Autodesk Inventor part; units mm, degrees
ref_plane "YZ Plane" through (0, 0, 0) normal (1, 0, 0) x (0, 1, 0)
ref_plane "XZ Plane" through (0, 0, 0) normal (0, 1, 0) x (-1, 0, 0)
ref_plane "XY Plane" through (0, 0, 0) normal (0, 0, 1) x (1, 0, 0)
sketch "Sketch1" plane through (0, 0, 0) normal (0, 0, 1) x (1, 0, 0)
  line L0 (-23.6137, 0) -> (-23.6137, 203.2)
  line L1 (-23.6137, 203.2) -> (484.3863, 203.2)
  line L2 (484.3863, 203.2) -> (484.3863, 279.4)
  line L3 (484.3863, 279.4) -> (1500.3863, 279.4)
  line L4 (1500.3863, 279.4) -> (1500.3863, 203.2)
  line L5 (1500.3863, 203.2) -> (2008.3863, 203.2)
  line L6 (2008.3863, 203.2) -> (2008.3863, 0)
  line L7 (2008.3863, 0) -> (-23.6137, 0)
  point P0 (0, 0)
  dimension "d0" = 203.2
  dimension "d1" = 508
  dimension "d2" = 76.2
  dimension "d3" = 1016
  dimension "d4" = 76.2
  dimension "d5" = 508
revolve "Revolution1" add sketch "Sketch1" angle 360 about axis through (2008.3863, 0, 0) along (-1, 0, 0)
chamfer "Chamfer1" distance 50.8 angle 45 2 edges at (-23.6137, -203.2, 0) (2008.3863, -203.2, 0)
properties part number "axle"
Work out the finished part from the listing and answer in its coordinate system (mm). A direction names the side the tool comes from. Coordinates: 2 decimals unless noted, no trailing zeros. Write each loop counter-clockwise with the first axis right and the second up, starting at its lowest first coordinate (ties: lowest second). Pieces come first, ordered by that corner, then holes. Notation, with made-up numbers: M 88,53 L 121,53 A16 cw 121,83 Z; hole C 44.25,80 d5. An arc over 180 degrees is marked long. Use one line per item in the form item = value. Start each with the question number.
1. The part is cut by section D-D (x = 897.5). Give the vertices of the cut face in (y, z).
2. Each of these flat-tipped pins is pushed along its axis until it touches: P1, Ø1.5, axis at x = 563, z = -153.5, coming from the +Y side; P2, Ø2, axis at y = -40, z = -207, coming from the -X side; P3, Ø8, axis at y = 64.5, z = -173.5, coming from the -X side. Where does it stop, or does it pass through?
3. Straight lines are drawn through the part: probe 1 along X at (y, z) = (-227.5, 116); probe 2 along X at (y, z) = (39, -170); probe 3 along Y at (x, z) = (1513.5, -188). For each, find the intervals that lie inside material, in ascending order. Write a range as from..to.
4. The part is cut by section C-C (x = 214). Give the vertices of the cut face in (y, z), plus the area to 3 significant figures.
5. The part is cut by section A-A (z = 0). Give the vertices of the cut face in (x, y), plus the area to 3 significant figures.
6. A tool of negligible diameter and unlimited length cuts with its end or side. For faces 1 (the face through (-23.614, -2, -2)), 2 (the face through (1732.187, -44.05, -198.368)), 3 (the face through (258.987, -44.05, -198.368)), from which of +Z, -Z, +X, -X, +Y, -Y can it reach the whole face along a straight path? Write none if from no direction.
Evaluation:
q1.outline = C 0,0 d558.8
q2.P1 = 233.95
q2.P2 = 484.39
q2.P3 = 5.09
q3.probe_1 = 484.39..1500.39
q3.probe_2 = -1.6..1986.37
q3.probe_3 = -77.11..77.11
q4.outline = C 0,0 d406.4
q4.area = 130,000 mm^2
q5.outline = M -23.61,-152.4 L 27.19,-203.2 L 484.39,-203.2 L 484.39,-279.4 L 1500.39,-279.4 L 1500.39,-203.2 L 1957.59,-203.2 L 2008.39,-152.4 L 2008.39,152.4 L 1957.59,203.2 L 1500.39,203.2 L 1500.39,279.4 L 484.39,279.4 L 484.39,203.2 L 27.19,203.2 L -23.61,152.4 Z
q5.area = 975,000 mm^2
q6.face_1 = +Z, -Z, -X, +Y, -Y
q6.face_2 = +X
q6.face_3 = -X
